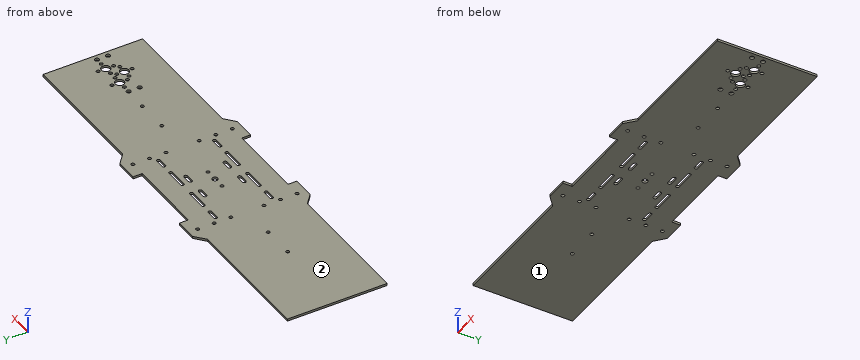
from build123d import *

# Parameters (mm, degrees)
SKETCH_1_R      = 1.55
SKETCH_1_R_2    = 2
SKETCH_1_R_3    = 4
SKETCH_1_R_4    = 2.5
EXTRUDE_1_DEPTH = 2


with BuildPart() as part:
    # 草图1 → 凸台-拉伸1 (new body)
    with BuildSketch(Plane.XY):
        Polygon((-35, 45), (35, 45), (35, 53.2), (55, 53.2), (64.431194454, 45), (185, 45), (185, -45), (64.431194454, -45), (55, -53.2), (35, -53.2), (35, -45), (-35, -45), (-35, -53.2), (-55, -53.2), (-64.431194454, -45), (-185, -45), (-185, 45), (-73.862388908, 45), (-64.431194454, 45), (-55, 53.2), (-35, 53.2), align=None)
        with Locations((49, -30)):
            Circle(SKETCH_1_R, mode=Mode.SUBTRACT)
        with Locations((49, -15)):
            Circle(SKETCH_1_R, mode=Mode.SUBTRACT)
        with Locations((10.5, 0)):
            Circle(SKETCH_1_R, mode=Mode.SUBTRACT)
        with Locations((-10.5, 0)):
            Circle(SKETCH_1_R, mode=Mode.SUBTRACT)
        with Locations((-49, -15)):
            Circle(SKETCH_1_R, mode=Mode.SUBTRACT)
        with Locations((-49, -30)):
            Circle(SKETCH_1_R, mode=Mode.SUBTRACT)
        with Locations((-49, 45)):
            Circle(SKETCH_1_R, mode=Mode.SUBTRACT)
        with Locations((49, 45)):
            Circle(SKETCH_1_R, mode=Mode.SUBTRACT)
        with Locations((-49, 30)):
            Circle(SKETCH_1_R, mode=Mode.SUBTRACT)
        with Locations((-49, 15)):
            Circle(SKETCH_1_R, mode=Mode.SUBTRACT)
        with Locations((49, 15)):
            Circle(SKETCH_1_R, mode=Mode.SUBTRACT)
        with Locations((49, 30)):
            Circle(SKETCH_1_R, mode=Mode.SUBTRACT)
        with Locations((49, -45)):
            Circle(SKETCH_1_R, mode=Mode.SUBTRACT)
        with Locations((-49, -45)):
            Circle(SKETCH_1_R, mode=Mode.SUBTRACT)
        with Locations((-80.5, 0)):
            Circle(SKETCH_1_R, mode=Mode.SUBTRACT)
        with Locations((-110, 0)):
            Circle(SKETCH_1_R, mode=Mode.SUBTRACT)
        with Locations((80.5, 0)):
            Circle(SKETCH_1_R, mode=Mode.SUBTRACT)
        with Locations((110, 0)):
            Circle(SKETCH_1_R, mode=Mode.SUBTRACT)
        with Locations((132, -0.8)):
            Circle(SKETCH_1_R_2, mode=Mode.SUBTRACT)
        with Locations((132, -10.8)):
            Circle(SKETCH_1_R_2, mode=Mode.SUBTRACT)
        with Locations((145.5, -0.8)):
            Circle(SKETCH_1_R_3, mode=Mode.SUBTRACT)
        with Locations((145.5, 6.2)):
            Circle(SKETCH_1_R, mode=Mode.SUBTRACT)
        with Locations((138.5, -0.8)):
            Circle(SKETCH_1_R, mode=Mode.SUBTRACT)
        with Locations((152.5, -0.8)):
            Circle(SKETCH_1_R, mode=Mode.SUBTRACT)
        with Locations((145.5, -7.8)):
            Circle(SKETCH_1_R, mode=Mode.SUBTRACT)
        with Locations((149, -11.3)):
            Circle(SKETCH_1_R, mode=Mode.SUBTRACT)
        with Locations((156, -4.3)):
            Circle(SKETCH_1_R, mode=Mode.SUBTRACT)
        with Locations((180, -10.8)):
            Circle(SKETCH_1_R_2, mode=Mode.SUBTRACT)
        with Locations((180, -0.8)):
            Circle(SKETCH_1_R_2, mode=Mode.SUBTRACT)
        with Locations((156, -18.3)):
            Circle(SKETCH_1_R, mode=Mode.SUBTRACT)
        with Locations((163, -11.3)):
            Circle(SKETCH_1_R, mode=Mode.SUBTRACT)
        with Locations((156, -11.3)):
            Circle(SKETCH_1_R_3, mode=Mode.SUBTRACT)
        with Locations((166.5, -0.8)):
            Circle(SKETCH_1_R_3, mode=Mode.SUBTRACT)
        with Locations((159.5, -0.8)):
            Circle(SKETCH_1_R, mode=Mode.SUBTRACT)
        with Locations((166.5, -7.8)):
            Circle(SKETCH_1_R, mode=Mode.SUBTRACT)
        with Locations((173.5, -0.8)):
            Circle(SKETCH_1_R, mode=Mode.SUBTRACT)
        with Locations((166.5, 6.2)):
            Circle(SKETCH_1_R, mode=Mode.SUBTRACT)
        Circle(SKETCH_1_R_4, mode=Mode.SUBTRACT)
        with BuildLine():
            Line((7.5, -16.25), (14.5, -16.25))
            ThreePointArc((14.5, -16.25), (16.05, -17.8), (14.5, -19.35))
            Line((14.5, -19.35), (7.5, -19.35))
            ThreePointArc((7.5, -19.35), (5.95, -17.8), (7.5, -16.25))
        make_face(mode=Mode.SUBTRACT)
        with BuildLine():
            Line((7, -23.85), (24.5, -23.85))
            ThreePointArc((24.5, -23.85), (26.05, -25.4), (24.5, -26.95))
            Line((24.5, -26.95), (7, -26.95))
            ThreePointArc((7, -26.95), (5.45, -25.4), (7, -23.85))
        make_face(mode=Mode.SUBTRACT)
        with BuildLine():
            Line((35, -23.85), (43, -23.85))
            ThreePointArc((43, -23.85), (44.55, -25.4), (43, -26.95))
            Line((43, -26.95), (35, -26.95))
            ThreePointArc((35, -26.95), (33.45, -25.4), (35, -23.85))
        make_face(mode=Mode.SUBTRACT)
        with BuildLine():
            Line((-35, -23.85), (-43, -23.85))
            ThreePointArc((-43, -23.85), (-44.55, -25.4), (-43, -26.95))
            Line((-43, -26.95), (-35, -26.95))
            ThreePointArc((-35, -26.95), (-33.45, -25.4), (-35, -23.85))
        make_face(mode=Mode.SUBTRACT)
        with BuildLine():
            Line((-7, -23.85), (-24.5, -23.85))
            ThreePointArc((-24.5, -23.85), (-26.05, -25.4), (-24.5, -26.95))
            Line((-24.5, -26.95), (-7, -26.95))
            ThreePointArc((-7, -26.95), (-5.45, -25.4), (-7, -23.85))
        make_face(mode=Mode.SUBTRACT)
        with BuildLine():
            Line((-7.5, -16.25), (-14.5, -16.25))
            ThreePointArc((-14.5, -16.25), (-16.05, -17.8), (-14.5, -19.35))
            Line((-14.5, -19.35), (-7.5, -19.35))
            ThreePointArc((-7.5, -19.35), (-5.95, -17.8), (-7.5, -16.25))
        make_face(mode=Mode.SUBTRACT)
        with BuildLine():
            Line((-7.5, 16.25), (-14.5, 16.25))
            ThreePointArc((-14.5, 16.25), (-16.05, 17.8), (-14.5, 19.35))
            Line((-14.5, 19.35), (-7.5, 19.35))
            ThreePointArc((-7.5, 19.35), (-5.95, 17.8), (-7.5, 16.25))
        make_face(mode=Mode.SUBTRACT)
        with BuildLine():
            Line((-7, 23.85), (-24.5, 23.85))
            ThreePointArc((-24.5, 23.85), (-26.05, 25.4), (-24.5, 26.95))
            Line((-24.5, 26.95), (-7, 26.95))
            ThreePointArc((-7, 26.95), (-5.45, 25.4), (-7, 23.85))
        make_face(mode=Mode.SUBTRACT)
        with BuildLine():
            Line((-35, 23.85), (-43, 23.85))
            ThreePointArc((-43, 23.85), (-44.55, 25.4), (-43, 26.95))
            Line((-43, 26.95), (-35, 26.95))
            ThreePointArc((-35, 26.95), (-33.45, 25.4), (-35, 23.85))
        make_face(mode=Mode.SUBTRACT)
        with BuildLine():
            Line((35, 23.85), (43, 23.85))
            ThreePointArc((43, 23.85), (44.55, 25.4), (43, 26.95))
            Line((43, 26.95), (35, 26.95))
            ThreePointArc((35, 26.95), (33.45, 25.4), (35, 23.85))
        make_face(mode=Mode.SUBTRACT)
        with BuildLine():
            Line((7, 23.85), (24.5, 23.85))
            ThreePointArc((24.5, 23.85), (26.05, 25.4), (24.5, 26.95))
            Line((24.5, 26.95), (7, 26.95))
            ThreePointArc((7, 26.95), (5.45, 25.4), (7, 23.85))
        make_face(mode=Mode.SUBTRACT)
        with BuildLine():
            Line((7.5, 16.25), (14.5, 16.25))
            ThreePointArc((14.5, 16.25), (16.05, 17.8), (14.5, 19.35))
            Line((14.5, 19.35), (7.5, 19.35))
            ThreePointArc((7.5, 19.35), (5.95, 17.8), (7.5, 16.25))
        make_face(mode=Mode.SUBTRACT)
    extrude(amount=EXTRUDE_1_DEPTH)


solid = part.part
Check sheet for the modelled part. Datum: model origin and axes. Units: mm. Face numbers are marked on the shaded views. Round coordinates to 2 decimals unless told otherwise and drop trailing zeros. Order: outer loops, then holes, each group sorted by start corner. A loop starts at its lowest first (then second) coordinate and runs counter-clockwise, first axis right, second up.
Q1. Cross-section at B-B, the plane z = 1.4. Give the number of separate pieces and of enclosed holes in the cut face, plus the area to 3 significant figures.
Filled sheet:
separate pieces: 1
enclosed holes: 50
area: 33,200 mm2
Q2. Draft check along Z on the marked faces 1 and 2. Enter one of: pulls with the +Z half, pulls with the -Z half, needs draft (parallel to the pull), parting line crosses it, or undercut.
Filled sheet:
face 1: pulls with the -Z half
face 2: pulls with the +Z half
Q3. Scan lines: L1, parallel to Y at x = 132, z = 1.2; L2, parallel to X at y = -17, z = 1.6; L3, parallel to Y at x = -36.5, z = 1.6. Record each from-to range of solid material in increasing order.
Filled sheet:
L1: y = -45 to -12.8, -8.8 to -2.8, 1.2 to 45
L2: x = -185 to -15.83, -6.17 to 6.17, 15.83 to 155.16, 156.84 to 185
L3: y = -53.2 to -26.95, -23.85 to 23.85, 26.95 to 53.2
Q4. Depth check by flat-ended pin: P1, Ø1.9, axis at x = -49, y = 30, coming from the +Z side; P2, Ø0.6, axis at x = 12, z = 1.5, coming from the -Y side. Enter the tip coordinate at first touch or a pass-through.
Filled sheet:
P1: passes through
P2: stops at y = -45
Q5. Cross-section at A-A, the plane x = 68. Enter the section's corners in (y, z), plus the area to 3 significant figures.
Filled sheet:
outline: (-45, 0) - (45, 0) - (45, 2) - (-45, 2) - close
area: 180 mm2
